```python
from build123d import *

# Parameters (mm, degrees)
SKETCH1_W           = 22.2758
SKETCH1_H           = 17.2085
BOSS_EXTRUDE1_DEPTH = 1.6256
SKETCH2_R           = 0.5715
CUT_EXTRUDE1_DEPTH  = 29.195501649
SKETCH3_W           = 1.524
SKETCH3_H           = 3.175
BOSS_EXTRUDE2_DEPTH = 1.905
SKETCH3_3_W         = 4.318
SKETCH3_3_H         = 2.54
BOSS_EXTRUDE3_DEPTH = 2.286
SKETCH3_4_W         = 4.572
SKETCH3_4_H         = 3.556
BOSS_EXTRUDE4_DEPTH = 1.27
SKETCH3_5_W         = 6.604
SKETCH3_5_H         = 6.604
BOSS_EXTRUDE5_DEPTH = 2.794
SKETCH3_6_R         = 1.397
BOSS_EXTRUDE6_DEPTH = 1.016
BOSS_EXTRUDE7_START = 0.254
SKETCH4_W           = 2.794
SKETCH4_H           = 5.334
SKETCH4_R           = 0.5715
BOSS_EXTRUDE7_DEPTH = 0.254


with BuildPart() as part:
    # Sketch1 → Boss-Extrude1 (new body)
    with BuildSketch(Plane.XY):
        with Locations((11.1379, 8.60425)):
            Rectangle(SKETCH1_W, SKETCH1_H)
    extrude(amount=BOSS_EXTRUDE1_DEPTH)

    # Sketch2 → Cut-Extrude1 (cut, through all)
    with BuildSketch(Plane.XY.offset(1.6256)):
        with Locations((1.8034, 15.46225)):
            Circle(SKETCH2_R)
        with Locations((1.8034, 12.92225)):
            Circle(SKETCH2_R)
        with Locations((20.4724, 15.46225)):
            Circle(SKETCH2_R)
        with Locations((20.4724, 12.92225)):
            Circle(SKETCH2_R)
        with Locations((20.4724, 4.28625)):
            Circle(SKETCH2_R)
        with Locations((20.4724, 1.74625)):
            Circle(SKETCH2_R)
        with Locations((1.8034, 4.28625)):
            Circle(SKETCH2_R)
        with Locations((1.8034, 1.74625)):
            Circle(SKETCH2_R)
    extrude(amount=-CUT_EXTRUDE1_DEPTH, mode=Mode.SUBTRACT)

    # Sketch3 → Boss-Extrude2 (add)
    with BuildSketch(Plane.XY.offset(1.6256)):
        with Locations((1.524, 8.60425)):
            Rectangle(SKETCH3_W, SKETCH3_H)
        with Locations((20.7518, 8.60425)):
            Rectangle(SKETCH3_W, SKETCH3_H)
    extrude(amount=BOSS_EXTRUDE2_DEPTH)

    # Sketch3_3 → Boss-Extrude3 (add)
    with BuildSketch(Plane.XY.offset(1.6256)):
        with Locations((6.477, 14.4145)):
            Rectangle(SKETCH3_3_W, SKETCH3_3_H)
    extrude(amount=BOSS_EXTRUDE3_DEPTH)

    # Sketch3_4 → Boss-Extrude4 (add)
    with BuildSketch(Plane.XY.offset(1.6256)):
        with Locations((7.366, 8.60425)):
            Rectangle(SKETCH3_4_W, SKETCH3_4_H)
    extrude(amount=BOSS_EXTRUDE4_DEPTH)

    # Sketch3_5 → Boss-Extrude5 (add)
    with BuildSketch(Plane.XY.offset(1.6256)):
        with Locations((15.4178, 10.8585)):
            Rectangle(SKETCH3_5_W, SKETCH3_5_H)
    extrude(amount=BOSS_EXTRUDE5_DEPTH)

    # Sketch3_6 → Boss-Extrude6 (add)
    with BuildSketch(Plane.XY.offset(1.6256)):
        with Locations(Location((16.1798, 2.032, 0), (0, 0, 180))):
            Circle(SKETCH3_6_R)
    extrude(amount=BOSS_EXTRUDE6_DEPTH)

    # Sketch4 → Boss-Extrude7 (add)
    # profile 1 of 4: a face of its own
    with BuildSketch(Plane.XY.offset(1.6256).offset(BOSS_EXTRUDE7_START)):
        with Locations((1.397, 14.5415)):
            Rectangle(SKETCH4_W, SKETCH4_H)
        with Locations((1.8034, 12.92225)):
            Circle(SKETCH4_R, mode=Mode.SUBTRACT)
        with Locations((1.8034, 15.46225)):
            Circle(SKETCH4_R, mode=Mode.SUBTRACT)
    # profile 2 of 4: a face of its own
    with BuildSketch(Plane.XY.offset(1.6256).offset(BOSS_EXTRUDE7_START)):
        with Locations((1.397, 2.667)):
            Rectangle(SKETCH4_W, SKETCH4_H)
        with Locations((1.8034, 1.74625)):
            Circle(SKETCH4_R, mode=Mode.SUBTRACT)
        with Locations((1.8034, 4.28625)):
            Circle(SKETCH4_R, mode=Mode.SUBTRACT)
    # profile 3 of 4: a face of its own
    with BuildSketch(Plane.XY.offset(1.6256).offset(BOSS_EXTRUDE7_START)):
        with Locations((20.8788, 2.667)):
            Rectangle(SKETCH4_W, SKETCH4_H)
        with Locations((20.4724, 4.28625)):
            Circle(SKETCH4_R, mode=Mode.SUBTRACT)
        with Locations((20.4724, 1.74625)):
            Circle(SKETCH4_R, mode=Mode.SUBTRACT)
    # profile 4 of 4: a face of its own
    with BuildSketch(Plane.XY.offset(1.6256).offset(BOSS_EXTRUDE7_START)):
        with Locations((20.8788, 14.5415)):
            Rectangle(SKETCH4_W, SKETCH4_H)
        with Locations((20.4724, 15.46225)):
            Circle(SKETCH4_R, mode=Mode.SUBTRACT)
        with Locations((20.4724, 12.92225)):
            Circle(SKETCH4_R, mode=Mode.SUBTRACT)
    extrude(amount=-BOSS_EXTRUDE7_DEPTH)


solid = part.part
```
Could you check a few things on this model? Use its own coordinates, in mm. A direction names the side the tool comes from. Round coordinates to 2 decimals unless told otherwise and drop trailing zeros. Order: outer loops, then holes, each group sorted by start corner. A loop starts at its lowest first (then second) coordinate and runs counter-clockwise, first axis right, second up. Notation, with made-up numbers: (38, -15) -> (90, -15) arc R6 ccw to (90, -6) -> close; hole circle Ø4 at (-3.75, 20). An arc over 180 degrees is marked (long way). One line per question, with ' | ' between items.
Q1. We'd pull the mould along X, two halves only. Please class faces 4 (the face through (6, 14, 3.912)), 5 (the face through (0, 8, 1)), 6 (the face through (1.232, 1.771, 0.953)): released by +X, released by -X, zero draft, split by the parting line, or undercut.
Computed values:
face 4: zero draft | face 5: released by -X | face 6: undercut
Q2. Which directions (+Z, -Z, +X, -X, +Y, -Y) give clear straight access to the entire face, cutting with the end or side of a thin tool? Please do faces 1 (the face through (7, 9, 2.896)), 2 (the face through (1, 3, 1.88)), 3 (the face through (7, 6.826, 2)).
Computed values:
face 1: +Z, -Y | face 2: +Z, -X, -Y | face 3: +Z, +X, -X, -Y
Q3. If I drill on line 1 (X direction, y = 1.75, z = 0.9); line 2 (X direction, y = 9, z = 2.85); line 3 (X direction, y = 7.25, z = 2.5), over which ranges is the centre line in solid material (lowest first)? Write a range as from..to.
Computed values:
line 1: 0..1.23, 2.37..19.9, 21.04..22.28 | line 2: 0.76..2.29, 5.08..9.65, 12.12..18.72, 19.99..21.51 | line 3: 0.76..2.29, 5.08..9.65, 19.99..21.51
Q4. I'm going to push flat-ended pins straight in: pin 1 (0.6 mm diameter, centred on y = 8.5, z = 2, fed in from +X); pin 2 (0.8 mm diameter, centred on x = 1.5, y = 14.5, fed in from +Z); pin 3 (1 mm diameter, centred on x = 7, z = 2.5, fed in from +Y). Where does each tip first touch, or does it pass through?
Computed values:
pin 1: x = 21.51 | pin 2: z = 1.88 | pin 3: y = 15.68
Q5. If we section it at C-C on x = 6.5: Write out the boundary of the cut face in (y, z).
Computed values:
outline: (0, 0) -> (17.21, 0) -> (17.21, 1.63) -> (15.68, 1.63) -> (15.68, 3.91) -> (13.14, 3.91) -> (13.14, 1.63) -> (10.38, 1.63) -> (10.38, 2.9) -> (6.83, 2.9) -> (6.83, 1.63) -> (0, 1.63) -> close
Q6. If we section it at A-A on z = 3.15: Write out the boundary of the cut face in (x, y), plus the area to 3 significant figures.
Computed values:
outline: (0.76, 7.02) -> (2.29, 7.02) -> (2.29, 10.19) -> (0.76, 10.19) -> close; (4.32, 13.14) -> (8.64, 13.14) -> (8.64, 15.68) -> (4.32, 15.68) -> close; (12.12, 7.56) -> (18.72, 7.56) -> (18.72, 14.16) -> (12.12, 14.16) -> close; (19.99, 7.02) -> (21.51, 7.02) -> (21.51, 10.19) -> (19.99, 10.19) -> close | area: 64.3 mm²
Q7. If we section it at B-B on y = 14.5: Write out the boundary of the cut face in (x, z), plus the area to 3 significant figures.
Computed values:
outline: (0, 0) -> (22.28, 0) -> (22.28, 1.88) -> (19.48, 1.88) -> (19.48, 1.63) -> (8.64, 1.63) -> (8.64, 3.91) -> (4.32, 3.91) -> (4.32, 1.63) -> (2.79, 1.63) -> (2.79, 1.88) -> (0, 1.88) -> close | area: 47.5 mm²
Q8. If we section it at D-D on z = 0.8: Give the number of separate pieces and of enclosed holes in the cut face, plus the area to 3 significant figures.
Computed values:
separate pieces: 1 | enclosed holes: 8 | area: 375 mm²
